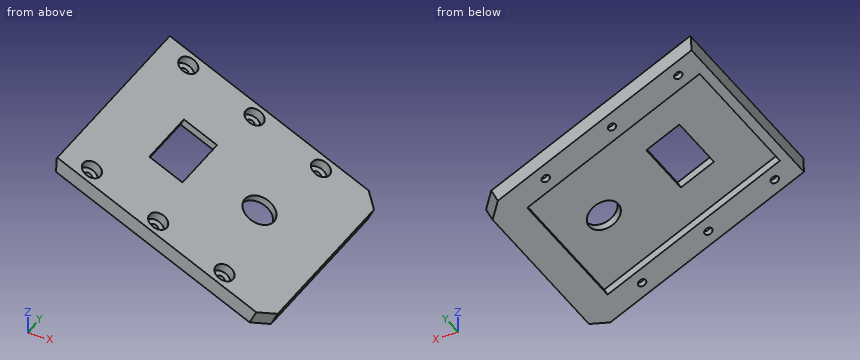
from build123d import *

# Parameters (mm, degrees)
PAD008_DEPTH            = 10
HOLE007_D               = 5.5
HOLE007_DEPTH           = 25
HOLE007_CBORE_D         = 13
HOLE007_CBORE_DEPTH     = 6.4
SKETCH024_W             = 130
SKETCH024_H             = 100
POCKET006_DEPTH         = 5
SKETCH025_W             = 25
SKETCH025_H             = 43
POCKET007_DEPTH         = 21
SKETCH026_R             = 11
POCKET008_DEPTH         = 12
PAD009_DEPTH            = 140
BODY004_PLACEMENT_ANGLE = 333.5


with BuildPart() as part:
    # Sketch022 → Pad008 (new body)
    with BuildSketch(Plane.XY):
        Polygon((0, 60), (0, -60), (-10, -70), (-156, -70), (-156, 70), (-10, 70), align=None)
    extrude(amount=PAD008_DEPTH)

    # Hole007
    with Locations(Plane.XY.offset(10)):
        with Locations((-140, 60), (-140, -60), (-90, -60), (-90, 60), (-40, 60), (-40, -60)):
            CounterBoreHole(HOLE007_D / 2, HOLE007_CBORE_D / 2, HOLE007_CBORE_DEPTH, depth=HOLE007_DEPTH)

    # Sketch024 → Pocket006 (cut)
    with BuildSketch(Plane.XY):
        with Locations((-85, 0)):
            Rectangle(SKETCH024_W, SKETCH024_H)
    extrude(amount=POCKET006_DEPTH, mode=Mode.SUBTRACT)

    # Sketch025 → Pocket007 (cut)
    with BuildSketch(Plane.XY):
        with Locations((-107.5, 0)):
            Rectangle(SKETCH025_W, SKETCH025_H)
    extrude(amount=POCKET007_DEPTH, mode=Mode.SUBTRACT)

    # Sketch026 → Pocket008 (cut)
    with BuildSketch(Plane.XY):
        with Locations((-50, 0)):
            Circle(SKETCH026_R)
    extrude(amount=POCKET008_DEPTH, mode=Mode.SUBTRACT)

    # Sketch027 → Pad009 (join)
    with BuildSketch(Plane.XZ.offset(70)):
        Polygon((-156, 10), (-160, 10), (-160, 9), (-156, 0), align=None)
    extrude(amount=-PAD009_DEPTH)


with BuildPart() as part_1:
    # Body004 placement: moved
    add(part.part.moved(Location((310, 0, 70))).rotate(Axis((310, 0, 70), (0, -1, 0)), BODY004_PLACEMENT_ANGLE))


solid = part_1.part
Source: CAD feature listing. Evaluate the final solid. Frame: model axes, mm. Give positions to 0.01 mm unless a question says otherwise; leave off trailing zeros. Write each loop counter-clockwise with the first axis right and the second up, starting at its lowest first coordinate (ties: lowest second). Pieces come first, ordered by that corner, then holes. Notation, with made-up numbers: (2.5, 2) -> (18.5, 2) arc R20 ccw to (18.5, 13) -> close; hole circle Ø3 at (73, 62). An arc over 180 degrees is marked (long way). Write item = value, one per line.
Q1. Cut plane D-D on x = 289.5. Return loops of the section in (y, z), then the cut area to 3 significant figures.
Here are the results:
outline = (-70, 80.22) -> (-50, 80.22) -> (-50, 85.81) -> (50, 85.81) -> (50, 80.22) -> (70, 80.22) -> (70, 91.39) -> (-70, 91.39) -> close
area = 1,010 mm²
Q2. Line query: line 1 (X direction, y = 57, z = 89); line 2 (Z direction, x = 273, y = -44); line 3 (X direction, y = -47, z = 100.5). Output: solid intervals per line, ascending. Write a range as from..to.
Here are the results:
line_1 = 271.89..279.96, 281.22..294.3
line_2 = 94.03..99.62
line_3 = 260.03..271.24
Q3. Cut plane A-A on y = 27. Return loops of the section in (x, z), then the cut area to 3 significant figures.
Here are the results:
outline = (170.39, 139.61) -> (175.76, 136.93) -> (177.99, 141.4) -> (294.33, 83.4) -> (292.1, 78.92) -> (310, 70) -> (314.46, 78.95) -> (171.27, 150.34) -> (170.83, 149.45) -> close
area = 932 mm²
Q4. First-contact query: pin 1 (4 mm diameter, centred on x = 259, z = 111, fed in from +Y); pin 2 (6 mm diameter, centred on y = -42, z = 94, fed in from +X); pin 3 (6 mm diameter, centred on y = 10, z = 111.5, fed in from +X). Flat tips, straight axial feed; report the tip coordinate or a pass-through.
Here are the results:
pin_1 = through
pin_2 = 290.29
pin_3 = 255.19
Q5. Cut plane B-B on x = 212. Return loops of the section in (y, z) (3 decimals).
Here are the results:
outline = (-70, 118.861) -> (-50, 118.861) -> (-50, 124.448) -> (-21.5, 124.448) -> (-21.5, 130.035) -> (-70, 130.035) -> close; (21.5, 124.448) -> (50, 124.448) -> (50, 118.861) -> (70, 118.861) -> (70, 130.035) -> (21.5, 130.035) -> close
Q6. Cut plane C-C on y = -5.5. Return loops of the section in (x, z), then the cut area to 3 significant figures.
Here are the results:
outline = (170.39, 139.61) -> (175.76, 136.93) -> (177.99, 141.4) -> (204.84, 128.02) -> (207.07, 132.49) -> (171.27, 150.34) -> (170.83, 149.45) -> close; (227.21, 116.86) -> (258.96, 101.04) -> (261.19, 105.51) -> (229.44, 121.34) -> close; (276.01, 92.53) -> (294.33, 83.4) -> (292.1, 78.92) -> (310, 70) -> (314.46, 78.95) -> (278.24, 97.01) -> close
area = 712 mm²
